Design review of the part built by this model. Coordinates are the model's own, in mm. A direction names the side the tool comes from. Give positions to 0.01 mm unless a question says otherwise; leave off trailing zeros. Order: outer loops, then holes, each group sorted by start corner. A loop starts at its lowest first (then second) coordinate and runs counter-clockwise, first axis right, second up. Notation, with made-up numbers: (58.5, -28.5) -> (89.5, -28.5) arc R13 ccw to (89.5, -15.5) -> close; hole circle Ø9 at (62.25, -6.5). An arc over 180 degrees is marked (long way). One line per item, written item: value.
from build123d import *

# Parameters (mm, degrees)
HEAD_START       = -3
SKETCH1_R        = 2.8
HEAD_DEPTH       = 3
SKETCH2_R        = 1.5
SHANK_DEPTH      = 8
HEX_START        = -3.2
HEX_SOCKET_DEPTH = 1.8


with BuildPart() as part:
    # Sketch1 → Head (new body)
    with BuildSketch(Plane.XY.offset(HEAD_START)):
        Circle(SKETCH1_R)
    extrude(amount=HEAD_DEPTH)

    # Sketch2 → Shank (add)
    with BuildSketch(Plane.XY):
        Circle(SKETCH2_R)
    extrude(amount=SHANK_DEPTH)

    # Sketch3 → Hex socket (cut)
    with BuildSketch(Plane.XY.offset(HEX_START)):
        Polygon((1.25, 0.721687836), (0, 1.443375673), (-1.25, 0.721687836), (-1.25, -0.721687836), (0, -1.443375673), (1.25, -0.721687836), align=None)
    extrude(amount=HEX_SOCKET_DEPTH, mode=Mode.SUBTRACT)


solid = part.part
Item 1: Add section B-B on x = 0.95. Give the boundary of the cut face in (y, z).
Returned:
outline: (-2.63, -3) -> (-0.89, -3) -> (-0.89, -1.4) -> (0.89, -1.4) -> (0.89, -3) -> (2.63, -3) -> (2.63, 0) -> (1.16, 0) -> (1.16, 8) -> (-1.16, 8) -> (-1.16, 0) -> (-2.63, 0) -> close
Item 2: Add section A-A on y = 0. Give the boundary of the cut face in (x, z), plus the area to 3 significant figures.
Returned:
outline: (-2.8, -3) -> (-1.25, -3) -> (-1.25, -1.4) -> (1.25, -1.4) -> (1.25, -3) -> (2.8, -3) -> (2.8, 0) -> (1.5, 0) -> (1.5, 8) -> (-1.5, 8) -> (-1.5, 0) -> (-2.8, 0) -> close
area: 36.8 mm²
Item 3: Add section C-C on z = -0.5. Give the boundary of the cut face in (x, y).
Returned:
outline: circle Ø5.6 at (0, 0)
Item 4: Add section D-D on z = 2.25. Give the boundary of the cut face in (x, y).
Returned:
outline: circle Ø3 at (0, 0)
Item 5: Machinability: for faces 4 (the flat face through (1.2, -1.2, 0)), 5 (the flat face through (-0.63, -1.08, -2.21)), 6 (the cylindrical face through (-2.8, 0.1, -1.5)), which of the approach directions +Z, -Z, +X, -X, +Y, -Y give a long, thin tool a straight path to every point of the face, cutting with its end or side? Answer none if there is none.
Returned:
face 4: +Z
face 5: -Z
face 6: +Z, -Z
Item 6: To check wall thickness, follow line 1 along Z through (x, y) = (0.95, -0.5); line 2 along X through (y, z) = (0.05, 2.5); line 3 along Z through (x, y) = (-1.35, -2.2). State the ranges of each line that lie inside material, in increasing order. Write a range as from..to.
Returned:
line 1: -1.4..8
line 2: -1.5..1.5
line 3: -3..0
Item 7: Clearance check with flat-ended pins moving along their axes: P1, Ø0.8, axis at x = -0.5, y = -0.5, coming from the -Z side; P2, Ø2, axis at y = -2, z = 4.5, coming from the +X side; P3, Ø1.6, axis at y = 0.5, z = -2, coming from the +X side. State where each tip first meets the part, or that it passes through.
Returned:
P1: z = -1.4
P2: x = 1.12
P3: x = 2.8
Item 8: Draft analysis for pull direction X (two halves, no side actions). For faces 1 (the flat face through (-1.25, 0, -2)), 2 (the cylindrical face through (-1.5, 0.07, 3.94)), 3 (the flat face through (0, 0, 8)), state which applies: pulls with the +X half, pulls with the -X half, needs draft (parallel to the pull), parting line crosses it, or undercut.
Returned:
face 1: undercut
face 2: parting line crosses it
face 3: needs draft
